```python
from build123d import *

# Parameters (mm, degrees)
BOSS_EXTRU_1_DEPTH                                = 5
FRAISAGE_POUR_T_TE_FRAIS_E_BOMB_E_M31_D           = 3.6
FRAISAGE_POUR_T_TE_FRAIS_E_BOMB_E_M31_CSINK_D     = 6.3
FRAISAGE_POUR_T_TE_FRAIS_E_BOMB_E_M31_CSINK_ANGLE = 90
ENL_V_MAT_EXTRU_1_DEPTH                           = 10


with BuildPart() as part:
    # Esquisse1 → Boss.-Extru.1 (new body)
    with BuildSketch(Plane(origin=(0, 0, 0), x_dir=(1, 0, 0), z_dir=(0, 1, 0))):
        with BuildLine():
            Line((-32.5, -10.256252677), (-117.5, -157.48057132))
            Line((-117.5, -157.48057132), (-169.461524227, -187.48057132))
            ThreePointArc((-169.461524227, -187.48057132), (-178.328455444, -230.127663943), (-136.961524227, -243.772222566))
            Line((-136.961524227, -243.772222566), (-85, -213.772222566))
            Line((-85, -213.772222566), (85, -213.772222566))
            Line((85, -213.772222566), (136.961524227, -243.772222566))
            ThreePointArc((136.961524227, -243.772222566), (178.328455444, -230.127663943), (169.461524227, -187.48057132))
            Line((169.461524227, -187.48057132), (117.5, -157.48057132))
            Line((117.5, -157.48057132), (32.5, -10.256252677))
            Line((32.5, -10.256252677), (32.5, 49.743747323))
            ThreePointArc((32.5, 49.743747323), (0, 78.746281322), (-32.5, 49.743747323))
            Line((-32.5, 49.743747323), (-32.5, -10.256252677))
        make_face()
        with BuildLine():
            ThreePointArc((-88.937370367, -203.535799534), (-92.731465593, -204.035301647), (-95.767497386, -201.705672515))
            Line((-95.767497386, -201.705672515), (-113.267497386, -171.394783383))
            ThreePointArc((-113.267497386, -171.394783383), (-113.766999499, -167.600688157), (-111.437370367, -164.564656364))
            Line((-111.437370367, -164.564656364), (-94.116862291, -154.564656364))
            ThreePointArc((-94.116862291, -154.564656364), (-90.322767066, -154.065154251), (-87.286735273, -156.394783383))
            Line((-87.286735273, -156.394783383), (-69.786735273, -186.705672515))
            ThreePointArc((-69.786735273, -186.705672515), (-69.28723316, -190.499767741), (-71.616862291, -193.535799534))
            Line((-71.616862291, -193.535799534), (-88.937370367, -203.535799534))
        make_face(mode=Mode.SUBTRACT)
        with BuildLine():
            ThreePointArc((71.616862291, -193.535799534), (69.28723316, -190.499767741), (69.786735273, -186.705672515))
            Line((69.786735273, -186.705672515), (87.286735273, -156.394783383))
            ThreePointArc((87.286735273, -156.394783383), (90.322767066, -154.065154251), (94.116862291, -154.564656364))
            Line((94.116862291, -154.564656364), (111.437370367, -164.564656364))
            ThreePointArc((111.437370367, -164.564656364), (113.766999499, -167.600688157), (113.267497386, -171.394783383))
            Line((113.267497386, -171.394783383), (95.767497386, -201.705672515))
            ThreePointArc((95.767497386, -201.705672515), (92.731465593, -204.035301647), (88.937370367, -203.535799534))
            Line((88.937370367, -203.535799534), (71.616862291, -193.535799534))
        make_face(mode=Mode.SUBTRACT)
        with BuildLine():
            Line((17.5, -35.964601431), (-17.5, -35.964601431))
            ThreePointArc((-17.5, -35.964601431), (-21.035533906, -34.500135337), (-22.5, -30.964601431))
            Line((-22.5, -30.964601431), (-22.5, -10.964601431))
            ThreePointArc((-22.5, -10.964601431), (-21.035533906, -7.429067525), (-17.5, -5.964601431))
            Line((-17.5, -5.964601431), (17.5, -5.964601431))
            ThreePointArc((17.5, -5.964601431), (21.035533906, -7.429067525), (22.5, -10.964601431))
            Line((22.5, -10.964601431), (22.5, -30.964601431))
            ThreePointArc((22.5, -30.964601431), (21.035533906, -34.500135337), (17.5, -35.964601431))
        make_face(mode=Mode.SUBTRACT)
    extrude(amount=BOSS_EXTRU_1_DEPTH)

    # Fraisage pour tête fraisée bombée M31 (through all)
    with Locations(Plane(origin=(18.169872981, 5, -4.564255399), x_dir=(0, 0, 1), z_dir=(0, 1, 0))):
        with Locations((0, 0), (181.304804312, -141.016123537), (213.336477965, -123.795670618), (0, -36.339745962), (181.088690368, 104.551604131), (213.336477965, 87.70428834)):
            CounterSinkHole(FRAISAGE_POUR_T_TE_FRAIS_E_BOMB_E_M31_D / 2, FRAISAGE_POUR_T_TE_FRAIS_E_BOMB_E_M31_CSINK_D / 2, counter_sink_angle=FRAISAGE_POUR_T_TE_FRAIS_E_BOMB_E_M31_CSINK_ANGLE)

    # Esquisse5 → Enlèv. mat.-Extru.1 (cut)
    with BuildSketch(Plane(origin=(0, 5, 0), x_dir=(1, 0, 0), z_dir=(0, 1, 0))):
        with BuildLine():
            Line((-117.5, -157.48057132), (-129.676377575, -178.570675931))
            Line((-129.676377575, -178.570675931), (-110.625797637, -213.772222566))
            Line((-110.625797637, -213.772222566), (-85, -213.772222566))
            add(Edge.make_bspline(
                [(-117.5, -157.48057132), (-151.940688813, -148.613043489), (-277.037698094, -222.560603045), (-150.450766074, -316.414471558), (-56.420377815, -257.105249939), (-85, -213.772222566)],
                knots=[0, 0, 0, 0, 0.411814668, 0.638484528, 1, 1, 1, 1], degree=3))
        make_face()
        with BuildLine():
            Line((-32.5, -10.256252677), (-20, 11.394382418))
            Line((-20, 11.394382418), (20, 11.394382418))
            Line((20, 11.394382418), (32.5, -10.256252677))
            add(Edge.make_bspline(
                [(0, 98.703141202), (74.821178569, 66.789103835), (32.5, -10.256252677)],
                knots=[0, 0, 0, 1, 1, 1], degree=2))
            add(Edge.make_bspline(
                [(0, 98.703141202), (-74.821178569, 66.789103835), (-32.5, -10.256252677)],
                knots=[0, 0, 0, 1, 1, 1], degree=2))
        make_face()
        with BuildLine():
            Line((117.5, -157.48057132), (129.676377575, -178.570675931))
            Line((129.676377575, -178.570675931), (110.625797637, -213.772222566))
            Line((110.625797637, -213.772222566), (85, -213.772222566))
            add(Edge.make_bspline(
                [(117.5, -157.48057132), (151.940688813, -148.613043489), (277.037698094, -222.560603045), (150.450766074, -316.414471558), (56.420377815, -257.105249939), (85, -213.772222566)],
                knots=[0, 0, 0, 0, 0.411814668, 0.638484528, 1, 1, 1, 1], degree=3))
        make_face()
    extrude(amount=-ENL_V_MAT_EXTRU_1_DEPTH, mode=Mode.SUBTRACT)


solid = part.part
```
Here's how the part is built. I have some questions about the finished solid (model axes, mm). A direction names the side the tool comes from. Round coordinates to 2 decimals unless told otherwise and drop trailing zeros. Order: outer loops, then holes, each group sorted by start corner. A loop starts at its lowest first (then second) coordinate and runs counter-clockwise, first axis right, second up. Notation, with made-up numbers: M -26,17 L -16,17 A25 cw -16,53 Z; hole C 5,-0.75 d2. An arc over 180 degrees is marked long. Answer as CSV lines item,"result".
Item 1: We'd pull the mould along X, two halves only. Please class faces 1 (the flat face through (78.414, 2.465, 171.762)), 2 (the flat face through (120.3, 2.5, 195.9)), 3 (the flat face through (-120.3, 2.5, 195.9)), 4 (the flat face through (-2, 5, 125)): +X half, -X half, draft (parallel to the pull), parting line (faces both ways), or undercut.
From the geometry:
face 1,"undercut"
face 2,"+X half"
face 3,"-X half"
face 4,"draft"
Item 2: Which directions (+Z, -Z, +X, -X, +Y, -Y) give clear straight access to the entire face, cutting with the end or side of a thin tool? Please do faces 5 (the flat face through (-2, 0, 125)), 6 (the flat face through (-80.16, 2.46, 198.47)).
From the geometry:
face 5,"+Z, -Z, +X, -X, -Y"
face 6,"+Y, -Y"
Item 3: Imagine slicing it at C-C on y = 2.6. Give the number of separate pieces and of enclosed holes in the cut face, and give its area (3 significant figures).
From the geometry:
separate pieces,"1"
enclosed holes,"9"
area,"32,800 mm2"
Item 4: Please list where these lines run through material, in increasing order: L1, parallel to X at y = 4.55, z = 188.5; L2, parallel to X at y = 0.35, z = 173; L3, parallel to Z at x = 102.5, y = 2.9. Write a range as [from, to].
From the geometry:
L1,"[-124.3, -103.39], [-69.17, 69.17], [103.39, 124.3]"
L2,"[-126.46, -112.34], [-77.7, 77.7], [112.34, 126.46]"
L3,"[131.5, 159.4], [190.04, 213.77]"
Item 5: Imagine slicing it at D-D on z = 49. List the corners of the cut face in (x, y) for me, and give its area (3 significant figures).
From the geometry:
outline,"M -54.87,0 L 54.87,0 L 54.87,5 L -54.87,5 Z"
area,"549 mm2"
Item 6: Imagine slicing it at B-B on x = 80.5. List the corners of the cut face in (y, z) for me, and give its area (3 significant figures).
From the geometry:
outline,"M 0,93.39 L 5,93.39 L 5,168.15 L 0,168.15 Z; M 0,198.66 L 5,198.66 L 5,213.77 L 0,213.77 Z"
area,"449 mm2"
Item 7: For pin 1 (6 mm diameter, centred on x = 105.87, z = 208.77, fed in from +Y); pin 2 (1.5 mm diameter, centred on y = 3, z = 22, fed in from +X); pin 3 (1.5 mm diameter, centred on y = 3, z = 25.5, fed in from -X), each with a flat end and sliding along its axis, tell me the tip position at first contact or that it passes through.
From the geometry:
pin 1,"y = 4.85"
pin 2,"x = 39.71"
pin 3,"x = -41.73"
Item 8: Imagine slicing it at A-A on x = -9. List the corners of the cut face in (y, z) for me.
From the geometry:
outline,"M 0,-11.39 L 5,-11.39 L 5,5.96 L 0,5.96 Z; M 0,35.96 L 5,35.96 L 5,213.77 L 0,213.77 Z"
